The model under review builds one solid part; all positions refer to its coordinate system, in mm. Face numbers are marked on the shaded views. A direction names the side the tool comes from. Give positions to 0.01 mm unless a question says otherwise; leave off trailing zeros. Write each loop counter-clockwise with the first axis right and the second up, starting at its lowest first coordinate (ties: lowest second). Pieces come first, ordered by that corner, then holes. Notation, with made-up numbers: (68, 33) - (75, 33) arc R8 ccw to (75, 47) - close; hole circle Ø11 at (-34.5, 87.5). An arc over 180 degrees is marked (long way). Write item = value, one per line.
```python
from build123d import *

# Parameters (mm, degrees)
SKETCH1_R           = 9
BODY_DEPTH          = 19
SKETCH2_R           = 4
BORE_DEPTH          = 12
SKETCH3_W           = 1.5
SKETCH3_H           = 9
BORE_FLAT_DEPTH     = 12
SKETCH4_R           = 3
MAGNET_POCKET_DEPTH = 3
SKETCH5_W           = 22
SKETCH5_H           = 14
ARM_SLOT_DEPTH      = 3
SKETCH6_R           = 1.25
ARM_SCREWS_DEPTH    = 6


with BuildPart() as part:
    # Sketch1 → Body (new body)
    with BuildSketch(Plane.XY):
        Circle(SKETCH1_R)
    extrude(amount=BODY_DEPTH)

    # Sketch2 → Bore (cut)
    with BuildSketch(Plane.XY):
        Circle(SKETCH2_R)
    extrude(amount=BORE_DEPTH, mode=Mode.SUBTRACT)

    # Sketch3 → Bore_flat (add)
    with BuildSketch(Plane.XY):
        with Locations((3.95, 0)):
            Rectangle(SKETCH3_W, SKETCH3_H)
    extrude(amount=BORE_FLAT_DEPTH)

    # Sketch4 → Magnet_pocket (cut)
    with BuildSketch(Plane.XY.offset(12)):
        Circle(SKETCH4_R)
    extrude(amount=MAGNET_POCKET_DEPTH, mode=Mode.SUBTRACT)

    # Sketch5 → Arm_slot (cut)
    with BuildSketch(Plane.XY.offset(16)):
        Rectangle(SKETCH5_W, SKETCH5_H)
    extrude(amount=ARM_SLOT_DEPTH, mode=Mode.SUBTRACT)

    # Sketch6 → Arm_screws (cut)
    with BuildSketch(Plane.XY.offset(10)):
        with Locations((-6, 0)):
            Circle(SKETCH6_R)
        with Locations((6, 0)):
            Circle(SKETCH6_R)
    extrude(amount=ARM_SCREWS_DEPTH, mode=Mode.SUBTRACT)


solid = part.part
```
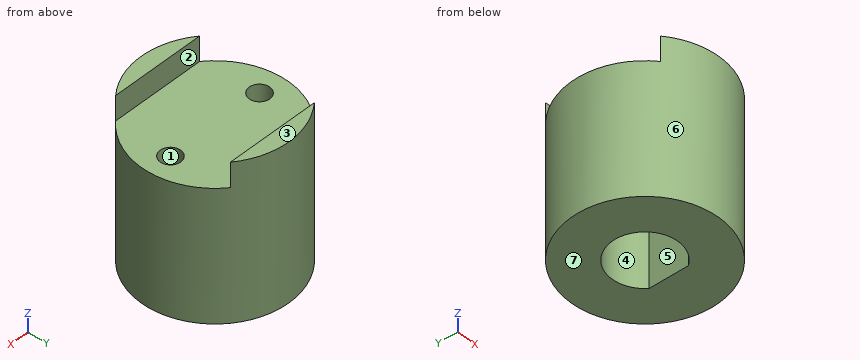
1. Machinability: for the marked faces 1, 2, 3 and 4, which of the approach directions +Z, -Z, +X, -X, +Y, -Y give a long, thin tool a straight path to every point of the face, cutting with its end or side? Answer none if there is none.
Findings below:
face_1 = +Z
face_2 = +Z, +X, -X
face_3 = +Z, +X, -X, +Y, -Y
face_4 = -Z
2. For line 1 (X direction, y = -1, z = 14.5); line 2 (Y direction, x = 0, z = 3.5); line 3 (Z direction, x = -4.25, y = -4.5), list the stretches that pass through material, from the lowest coordinate up. Write a range as from..to.
Findings below:
line_1 = -8.94..-6.75, -5.25..-2.83, 2.83..5.25, 6.75..8.94
line_2 = -9..-4, 4..9
line_3 = 0..16
3. Take a section at B-B on y = 0. Give the boundary of the cut face in (x, z).
Findings below:
outline = (-9, 0) - (-4, 0) - (-4, 12) - (-3, 12) - (-3, 15) - (3, 15) - (3, 12) - (3.2, 12) - (3.2, 0) - (9, 0) - (9, 16) - (7.25, 16) - (7.25, 10) - (4.75, 10) - (4.75, 16) - (-4.75, 16) - (-4.75, 10) - (-7.25, 10) - (-7.25, 16) - (-9, 16) - close
4. Insertion check: P1, Ø6, axis at y = -4, z = 13, coming from the +X side; P2, Ø1.8, axis at x = 0, y = 0, coming from the -Z side; P3, Ø5, axis at x = 0, y = 0, coming from the +Z side. Each pin has a flat end and moves straight along its axis. Give the tip position at first contact, or say it passes through.
Findings below:
P1 = 8.94
P2 = 15
P3 = 16
5. Take a section at D-D on z = 18. Give the boundary of the cut face in (x, y).
Findings below:
outline = (-5.66, -7) arc R9 ccw to (5.66, -7) - close; (-5.66, 7) - (5.66, 7) arc R9 ccw to start
6. Take a section at A-A on z = 11.25. Give the boundary of the cut face in (x, y), and give its area (3 significant figures).
Findings below:
outline = circle Ø18 at (0, 0); hole circle Ø2.5 at (-6, 0); hole (3.2, -2.4) - (3.2, 2.4) arc R4 ccw (long way) to start; hole circle Ø2.5 at (6, 0)
area = 197 mm²
7. Take a section at C-C on x = 0. Give the boundary of the cut face in (y, z), and give its area (3 significant figures).
Findings below:
outline = (-9, 0) - (-4, 0) - (-4, 12) - (-3, 12) - (-3, 15) - (3, 15) - (3, 12) - (4, 12) - (4, 0) - (9, 0) - (9, 19) - (7, 19) - (7, 16) - (-7, 16) - (-7, 19) - (-9, 19) - close
area = 186 mm²
8. Draft analysis for pull direction X (two halves, no side actions). For the marked faces 5, 6 and 7, state which applies: +X half, -X half, draft (parallel to the pull), parting line (faces both ways), or undercut.
Findings below:
face_5 = undercut
face_6 = parting line
face_7 = draft
